For this review, take the finished solid that the model builds, in its own axes (mm). A direction names the side the tool comes from. Coordinates: 2 decimals unless noted, no trailing zeros. Write each loop counter-clockwise with the first axis right and the second up, starting at its lowest first coordinate (ties: lowest second). Pieces come first, ordered by that corner, then holes.
Autodesk Inventor part; units mm, degrees
ref_plane "YZ Plane" through (0, 0, 0) normal (1, 0, 0) x (0, 1, 0)
ref_plane "XZ Plane" through (0, 0, 0) normal (0, 1, 0) x (-1, 0, 0)
ref_plane "XY Plane" through (0, 0, 0) normal (0, 0, 1) x (1, 0, 0)
sketch "Sketch1" plane through (0, 0, 0) normal (0, 0, 1) x (1, 0, 0)
  circle A0 centre (0, 0) radius 3
  circle A1 centre (0, 0) radius 5.25
  dimension "d0" = 6
  dimension "d1" = 10.5
extrude "Extrusion1" add sketch "Sketch1" along normal blind 0.8
extrude "Extrusion2" add sketch "Sketch1" along normal blind 16.8 contours A0
thread "Thread1"
sketch "Boceto3" plane through (0, 0, 0) normal (0, 0, -1) x (-1, 0, 0)
  circle A0 centre (0, 0) radius 5.25
extrude "Extrusión3" add sketch "Boceto3" along normal blind 2.5
fillet "Empalme2" radius 2.5 1 edges at (5.25, 0, -2.5)
sketch "Boceto4" plane through (0, 0, -2.5) normal (0, 0, -1) x (-1, 0, 0)
  line L0 (-2.2122, -1.978) -> (-2.8191, 0.9269)
  line L1 (-2.8191, 0.9269) -> (-0.6069, 2.9049)
  line L2 (-0.6069, 2.9049) -> (2.2122, 1.978)
  line L3 (2.2122, 1.978) -> (2.8191, -0.9269)
  line L4 (2.8191, -0.9269) -> (0.6069, -2.9049)
  line L5 (0.6069, -2.9049) -> (-2.2122, -1.978)
  point P0 (0, 0)
  point P1 (0, 0)
  dimension "d12" = 5.14
extrude "Extrusión4" cut sketch "Boceto4" against normal blind 2.5
chamfer "Chaflán1" distance 0.2 angle 45 1 edges at (-3, 0, 16.8)
properties part number "Tornillo Allen cabeza botón M6x16mm"
1) Tool access review of faces 4 (the face through (0.78, -2.45, -1.27)), 5 (the face through (2.3, -2.3, 0.8)): name each direction out of +Z, -Z, +X, -X, +Y, -Y from which nothing blocks a thin tool from reaching the whole face with its end or side.
2) Consider section A-A (y = 0). Give the boundary of the cut face in (x, z), then the cut area to 3 significant figures.
3) Consider section C-C (z = -0.5). Give the boundary of the cut face in (x, y).
4) Consider section B-B (z = 6.75). Give the boundary of the cut face in (x, y).
5) For L1, parallel to Z at x = -1.25, y = 3; L2, parallel to Z at x = 0, y = -0.75; L3, parallel to X at y = 2.25, z = 6, list the stretches that pass through material, from the lowest coordinate up.
6) Clearance check with flat-ended pins moving along their axes: P1, Ø2, axis at x = -4, y = 3, coming from the +Z side; P2, Ø1.5, axis at x = -1.5, z = 1, coming from the -Y side; P3, Ø2, axis at x = 3.5, z = 4.5, coming from the +Y side. State where each tip first meets the part, or that it passes through.
7) The part is to be moulded in two halves that separate along Y. For faces 1 (the face through (-3, 0, 9)), 2 (the face through (0, 0, 16.8)), 3 (the face through (2.51, -0.55, -1.27)), say which applies: pulls with the +Y half, pulls with the -Y half, needs draft (parallel to the pull), parting line crosses it, or undercut.
Results:
1. face 4: -Z
1. face 5: +Z
2. outline: (-5.25, 0) arc R2.5 ccw to (-2.75, -2.5) - (-2.63, -2.5) - (-2.63, 0) - (2.63, 0) - (2.63, -2.5) - (2.75, -2.5) arc R2.5 ccw to (5.25, 0) - (5.25, 0.8) - (3, 0.8) - (3, 16.6) - (2.8, 16.8) - (-2.8, 16.8) - (-3, 16.6) - (-3, 0.8) - (-5.25, 0.8) - close
2. area: 115 mm2
3. outline: circle Ø10.4 at (0, 0); hole (-2.82, -0.93) - (-0.61, -2.9) - (2.21, -1.98) - (2.82, 0.93) - (0.61, 2.9) - (-2.21, 1.98) - close
4. outline: circle Ø6 at (0, 0)
5. L1: z = -2.45 to 0.8
5. L2: z = 0 to 16.8
5. L3: x = -1.98 to 1.98
6. P1: stops at z = 0.8
6. P2: stops at y = -5.19
6. P3: stops at y = 1.66
7. face 1: parting line crosses it
7. face 2: needs draft
7. face 3: undercut
